from build123d import *

# Parameters (mm, degrees)
F0_W        = 139.7
F0_H        = 63.5
F1_DEPTH    = 19.05
F2_W        = 134.62
F2_H        = 58.42
F3_DEPTH    = 35.56
F4_R        = 1.5875
F5_DEPTH    = 2.54
F6_R        = 4.3815
F6_R_2      = 1.5875
F7_DEPTH    = 2.54
F8_W        = 6.35
F8_H        = 6.35
F9_DEPTH    = 12.7
F10_SIZE2   = 7.567625
F10_SIZE    = 6.34999
F10_2_SIZE2 = 7.567625
F10_2_SIZE  = 6.34999
F11_SIZE2   = 7.567625
F11_SIZE    = 6.34999
F11_2_SIZE2 = 7.567625
F11_2_SIZE  = 6.34999
F12_R       = 1.143
F13_DEPTH   = 12.7


# Not quite as in the source:
# - a fillet or chamfer is up to 0.001 mm smaller than in the source, because OpenCascade refuses the exact size


with BuildPart() as f1:
    # F0 (on Top) → F1 (new body, symmetric)
    with BuildSketch(Plane.XY):
        Rectangle(F0_W, F0_H)
    extrude(amount=F1_DEPTH, both=True)

    # F2 (on face) → F3 (cut)
    with BuildSketch(Plane.XY.offset(19.05)):
        Rectangle(F2_W, F2_H)
    extrude(amount=-F3_DEPTH, mode=Mode.SUBTRACT)

    # F4 (on face) → F5 (cut, through all)
    with BuildSketch(Plane.XZ.offset(31.75)):
        with Locations((50.8, 0)):
            Circle(F4_R)
    extrude(amount=-F5_DEPTH, mode=Mode.SUBTRACT)

    # F6 (on face) → F7 (cut, through all)
    with BuildSketch(Plane(origin=(0, 31.75, 0), x_dir=(-1, 0, 0), z_dir=(0, 1, 0))):
        with Locations((-31.75, 0)):
            Circle(F6_R)
        with Locations((-6.35, 0)):
            Circle(F6_R)
        with Locations((19.05, 0)):
            Circle(F6_R)
        with Locations((50.8, 9.525)):
            Circle(F6_R_2)
        with Locations((38.1, 9.525)):
            Circle(F6_R_2)
        with Locations((57.15, -9.525)):
            Circle(F6_R)
        with Locations((38.1, -9.525)):
            Circle(F6_R)
        with Locations((-57.15, 0)):
            Circle(F6_R)
    extrude(amount=-F7_DEPTH, mode=Mode.SUBTRACT)

    # F8 (on face) → F9 (join)
    with BuildSketch(Plane.XY.offset(19.05)):
        with Locations((-64.135, -26.035)):
            Rectangle(F8_W, F8_H)
        with Locations((64.135, 26.035)):
            Rectangle(F8_W, F8_H)
        with Locations((64.135, -26.035)):
            Rectangle(F8_W, F8_H)
        with Locations((-64.135, 26.035)):
            Rectangle(F8_W, F8_H)
    extrude(amount=-F9_DEPTH)

    # F10 (size 6.35 and 7.567635313 in the source; OpenCascade refuses exactly that, so slightly less here)
    f10_edges = [f1.edges().sort_by_distance(p)[0] for p in [
        (-60.96, 26.035, 6.35),
    ]]
    f10_side = f1.faces().sort_by_distance((-64.135, 26.035, 6.35))[0]
    chamfer(f10_edges, length=F10_SIZE, length2=F10_SIZE2, reference=f10_side)

    # F10#2 (size 6.35 and 7.567635313 in the source; OpenCascade refuses exactly that, so slightly less here)
    f10_2_edges = [f1.edges().sort_by_distance(p)[0] for p in [
        (60.96, -26.035, 6.35),
    ]]
    f10_2_side = f1.faces().sort_by_distance((64.135, -26.035, 6.35))[0]
    chamfer(f10_2_edges, length=F10_2_SIZE, length2=F10_2_SIZE2, reference=f10_2_side)

    # F11 (size 6.35 and 7.567635313 in the source; OpenCascade refuses exactly that, so slightly less here)
    f11_edges = [f1.edges().sort_by_distance(p)[0] for p in [
        (60.96, 26.035, 6.35),
    ]]
    f11_side = f1.faces().sort_by_distance((64.135, 26.035, 6.35))[0]
    chamfer(f11_edges, length=F11_SIZE, length2=F11_SIZE2, reference=f11_side)

    # F11#2 (size 6.35 and 7.567635313 in the source; OpenCascade refuses exactly that, so slightly less here)
    f11_2_edges = [f1.edges().sort_by_distance(p)[0] for p in [
        (-60.96, -26.035, 6.35),
    ]]
    f11_2_side = f1.faces().sort_by_distance((-64.135, -26.035, 6.35))[0]
    chamfer(f11_2_edges, length=F11_2_SIZE, length2=F11_2_SIZE2, reference=f11_2_side)

    # F12 (on face) → F13 (cut)
    with BuildSketch(Plane.XY.offset(19.05)):
        with Locations((-64.135, 26.035)):
            Circle(F12_R)
        with Locations((64.135, 26.035)):
            Circle(F12_R)
        with Locations((-64.135, -26.035)):
            Circle(F12_R)
        with Locations((64.135, -26.035)):
            Circle(F12_R)
    extrude(amount=-F13_DEPTH, mode=Mode.SUBTRACT)


solid = f1.part
Source: CAD feature listing. Evaluate the final solid. Frame: model axes, mm. A direction names the side the tool comes from. Give positions to 0.01 mm unless a question says otherwise; leave off trailing zeros. Write each loop counter-clockwise with the first axis right and the second up, starting at its lowest first coordinate (ties: lowest second). Pieces come first, ordered by that corner, then holes. Notation, with made-up numbers: (-3.75, -23.75) -> (35.25, -23.75) arc R25 cw to (35.25, -1.75) -> close; hole circle Ø8 at (-35, 81). An arc over 180 degrees is marked (long way). Return JSON: item names as keys, results as strings. Group by question number.
1. Section A-A, the plane x = 50.8. Output: boundary loops of the cut face in (y, z), then the cut area to 3 significant figures.
2. Pin query (flat end, axial travel): pin 1 Ø2 at (x, y) = (43, -24.5) entering from +Z. Return the tip coordinate at first contact, or that it passes through.
3. Access query for faces 5 (the face through (-42.15, 30.5, -11.2)), 6 (the face through (-65, 22.86, 14)), 7 (the face through (64.09, 27.4, 10.19)), 8 (the face through (49.214, -30.498, 0.07)). Directions: +Z, -Z, +X, -X, +Y, -Y. A direction counts if a zero-diameter tool reaches every point of the face in a straight line with its end or side. Return the directions, or none.
4. Material intervals for line 1 (Z direction, x = -38.1, y = 30.05); line 2 (Y direction, x = -62, z = 14); line 3 (Y direction, x = -12.5, z = 17), sorted ascending. Write a range as from..to.
5. Mould query, pull axis X, two halves, no side actions, for faces 1 (the face through (69.85, 0, 0)), 2 (the face through (64.09, -27.49, 10.19)), 3 (the face through (-16, -30, 19.05)), 4 (the face through (-69.85, 0, 0)). Classes: +X half, -X half, draft (parallel to the pull), parting line (faces both ways), or undercut.
6. Section C-C, the plane y = -16. Output: boundary loops of the cut face in (x, z), then the cut area to 3 significant figures.
7. Section B-B, the plane z = 0. Output: boundary loops of the cut face in (x, y).
8. Section D-D, the plane x = -38.1. Output: boundary loops of the cut face in (y, z), then the cut area to 3 significant figures.
Determined:
{
 "1": {"outline": "(-31.75, -19.05) -> (31.75, -19.05) -> (31.75, 19.05) -> (29.21, 19.05) -> (29.21, -16.51) -> (-29.21, -16.51) -> (-29.21, -1.59) -> (-31.75, -1.59) -> close; (-31.75, 1.59) -> (-29.21, 1.59) -> (-29.21, 19.05) -> (-31.75, 19.05) -> close", "area": "334 mm2"},
 "2": {"pin 1": "stops at z = -16.51"},
 "3": {"face 5": "+Y", "face 6": "+Z", "face 7": "none", "face 8": "-Y"},
 "4": {"line 1": "z = -19.05..-13.91, -5.14..7.94, 11.11..19.05", "line 2": "y = -31.75..-22.86, 22.86..31.75", "line 3": "y = -31.75..-29.21, 29.21..31.75"},
 "5": {"face 1": "+X half", "face 2": "undercut", "face 3": "draft", "face 4": "-X half"},
 "6": {"outline": "(-69.85, -19.05) -> (69.85, -19.05) -> (69.85, 19.05) -> (67.31, 19.05) -> (67.31, -16.51) -> (-67.31, -16.51) -> (-67.31, 19.05) -> (-69.85, 19.05) -> close", "area": "535 mm2"},
 "7": {"outline": "(-69.85, -31.75) -> (49.21, -31.75) -> (49.21, -29.21) -> (-67.31, -29.21) -> (-67.31, 29.21) -> (-23.43, 29.21) -> (-23.43, 31.75) -> (-69.85, 31.75) -> close; (-14.67, 29.21) -> (1.97, 29.21) -> (1.97, 31.75) -> (-14.67, 31.75) -> close; (10.73, 29.21) -> (27.37, 29.21) -> (27.37, 31.75) -> (10.73, 31.75) -> close; (36.13, 29.21) -> (52.77, 29.21) -> (52.77, 31.75) -> (36.13, 31.75) -> close; (52.39, -31.75) -> (69.85, -31.75) -> (69.85, 31.75) -> (61.53, 31.75) -> (61.53, 29.21) -> (67.31, 29.21) -> (67.31, -29.21) -> (52.39, -29.21) -> close"},
 "8": {"outline": "(-31.75, -19.05) -> (31.75, -19.05) -> (31.75, -13.91) -> (29.21, -13.91) -> (29.21, -16.51) -> (-29.21, -16.51) -> (-29.21, 19.05) -> (-31.75, 19.05) -> close; (29.21, -5.14) -> (31.75, -5.14) -> (31.75, 7.94) -> (29.21, 7.94) -> close; (29.21, 11.11) -> (31.75, 11.11) -> (31.75, 19.05) -> (29.21, 19.05) -> close", "area": "312 mm2"}
}
